```python
from build123d import *

# Parameters (mm, degrees)
SKETCH3_W                = 30
SKETCH3_H                = 25
BASETOPPLANE_DEPTH       = 30
BOSS_EXTRUDE1_DEPTH      = 5
BOSS_EXTRUDE1_DEPTH_BACK = 27
SKETCH6_W                = 34
SKETCH6_H                = 20
CUT_EXTRUDE1_DEPTH       = 39.668462602
SKETCH7_W                = 15
SKETCH7_H                = 10
BACKBAR_DEPTH            = 60
SIDECONNECT_DEPTH        = 5
SIDECONNECT_DEPTH_BACK   = 17
SKETCH8_W                = 40
SKETCH8_H                = 15
SKETCH9_W                = 30
SKETCH9_H                = 25
SIDESLIDER_DEPTH         = 17.5
MOUNTINGCUT_DEPTH        = 88.316641384
DRILLFORMOVEMENT_D       = 10
SKETCH17_W               = 15
SKETCH17_H               = 15
FRONTBAR_DEPTH           = 50


with BuildPart() as part:
    # Sketch3 → baseTopPlane (new body)
    with BuildSketch(Plane(origin=(0, 0, 0), x_dir=(1, 0, 0), z_dir=(0, 1, 0))):
        Rectangle(SKETCH3_W, SKETCH3_H)
    extrude(amount=BASETOPPLANE_DEPTH)

    # Sketch6 → Boss-Extrude1 (add, two sides: drawn at the far end of the back side and taken through both)
    with BuildSketch(Plane.XY.offset(12.5).offset(-BOSS_EXTRUDE1_DEPTH_BACK)):
        with Locations((0, 14.294511799)):
            Rectangle(SKETCH6_W, SKETCH6_H)
    extrude(amount=BOSS_EXTRUDE1_DEPTH + BOSS_EXTRUDE1_DEPTH_BACK)

    # Sketch4 → Cut-Extrude1 (cut, through all)
    with BuildSketch(Plane(origin=(0, 30, 0), x_dir=(1, 0, 0), z_dir=(0, 1, 0))):
        with BuildLine():
            Line((0, -12.5), (10, -12.5))
            Line((10, -12.5), (8, -10.5))
            Line((8, -10.5), (8, -8.5))
            ThreePointArc((8, -8.5), (9.060660172, -8.060660172), (9.5, -7))
            ThreePointArc((9.5, -7), (9.646446609, -6.646446609), (10, -6.5))
            Line((10, -6.5), (10, -4.5))
            ThreePointArc((10, -4.5), (8.939339828, -4.060660172), (8.5, -3))
            ThreePointArc((8.5, -3), (8.353553391, -2.646446609), (8, -2.5))
            Line((8, -2.5), (0, -2.5))
            Line((0, -2.5), (0, -12.5))
        make_face()
    cut_extrude1 = extrude(amount=-CUT_EXTRUDE1_DEPTH, mode=Mode.SUBTRACT)

    # Mirror1: Cut-Extrude1 across plane
    add(cut_extrude1.mirror(Plane(origin=(0, 0, 2.5), x_dir=(0, 0, 1), z_dir=(-1, 0, 0))), mode=Mode.SUBTRACT)

    # Sketch7 → BackBar (add)
    with BuildSketch(Plane(origin=(0, 0, -14.5), x_dir=(-1, 0, 0), z_dir=(0, 0, -1))):
        with Locations((0, 14.294511799)):
            Rectangle(SKETCH7_W, SKETCH7_H)
    extrude(amount=BACKBAR_DEPTH)

    # Sketch8 → sideConnect (add, two sides: drawn at the far end of the back side and taken through both)
    with BuildSketch(Plane.ZY.offset(7.5).offset(-SIDECONNECT_DEPTH_BACK)):
        with Locations((-57.5, 14.294511799)):
            Rectangle(SKETCH8_W, SKETCH8_H)
    extrude(amount=SIDECONNECT_DEPTH + SIDECONNECT_DEPTH_BACK)

    # Sketch9 → sideSlider (add)
    with BuildSketch(Plane.ZY.offset(12.5)):
        with Locations((-57.5, 14.294511799)):
            Rectangle(SKETCH9_W, SKETCH9_H)
    extrude(amount=SIDESLIDER_DEPTH)

    # Sketch13 → mountingCut (cut, through all)
    with BuildSketch(Plane(origin=(0, 26.794511799, 0), x_dir=(1, 0, 0), z_dir=(0, 1, 0))):
        Polygon((-30, 64), (-30, 51), (-24.75, 51), (-23.5, 49.75), (-26.25, 49.75), (-26.25, 47.25), (-19.75, 47.25), (-19.75, 53.75), (-22.25, 53.75), (-22.25, 51.25), (-24.75, 53.75), (-24.75, 61.25), (-22.25, 63.75), (-22.25, 61.25), (-19.75, 61.25), (-19.75, 67.75), (-26.25, 67.75), (-26.25, 65.25), (-23.5, 65.25), (-24.75, 64), align=None)
    extrude(amount=-MOUNTINGCUT_DEPTH, mode=Mode.SUBTRACT)

    # DrillforMovement (through all)
    with Locations(Plane(origin=(0, 21.794511799, 0), x_dir=(1, 0, 0), z_dir=(0, 1, 0))):
        with Locations((0, 57.5)):
            Hole(DRILLFORMOVEMENT_D / 2)

    # Sketch17 → frontBar (add)
    with BuildSketch(Plane.XY.offset(17.5)):
        with Locations((0, 14.294511799)):
            Rectangle(SKETCH17_W, SKETCH17_H)
    extrude(amount=FRONTBAR_DEPTH)


solid = part.part
```
Here's how the part is built. I have some questions about the finished solid (model axes, mm). A direction names the side the tool comes from. Give positions to 0.01 mm unless a question says otherwise; leave off trailing zeros. Loops run counter-clockwise (first coordinate to the right, second up) from the corner with the lowest first, then second, coordinate; pieces in that order, holes last. Notation, with made-up numbers: M 37,22 L 41,22 A26 cw 41,49 Z; hole C 53.25,69.25 d4. An arc over 180 degrees is marked long. Return JSON: item names as keys, results as strings.
Item 1: On a 3-axis mill with a long thin cutter (end or side, diameter ignored), from which of +Z, -Z, +X, -X, +Y, -Y can I reach the whole of each face in a straight line? I mean faces 1 (the flat face through (0, 19.295, -26)), 2 (the flat face through (-27, 14, -51)), 3 (the flat face through (-6, 6.795, -58)), 4 (the flat face through (-19.75, 14, -50)). Say none if no direction works.
A:
{"face 1": "+X, -X, +Y", "face 2": "-X, +Y, -Y", "face 3": "-Z, +X, -Y", "face 4": "+Y, -Y"}
Item 2: Thinking about a two-plate mould opening in X: for faces 5 (the flat face through (12, 27, 12.5)), 6 (the flat face through (15, 27, 0)), 7 (the flat face through (-26.25, 14, -49)), 8 (the flat face through (-30, 14, -68)), which applies, released by +X, released by -X, zero draft, split by the parting line, or undercut?
A:
{"face 5": "zero draft", "face 6": "released by +X", "face 7": "undercut", "face 8": "released by -X"}
Item 3: I'm going to push flat-ended pins straight in: pin 1 Ø3.5 at (y, z) = (2.5, -4) entering from +X; pin 2 Ø1.5 at (x, y) = (12, 15.5) entering from -Z; pin 3 Ø7.5 at (x, z) = (3.5, 52) entering from -Y. Where does each tip first touch, or does it pass through?
A:
{"pin 1": "stops at x = 15", "pin 2": "stops at z = -14.5", "pin 3": "stops at y = 6.79"}
Item 4: Imagine slicing it at C-C on z = -3.5. List the corners of the cut face in (x, y) for me.
A:
{"outline": "M -17,4.29 L -15,4.29 L -15,0 L 15,0 L 15,4.29 L 17,4.29 L 17,24.29 L 15,24.29 L 15,30 L -15,30 L -15,24.29 L -17,24.29 Z"}
Item 5: Imagine slicing it at B-B on x = 0. List the corners of the cut face in (y, z) for me, then the cut area to 3 significant figures.
A:
{"outline": "M 0,-12.5 L 4.29,-12.5 L 4.29,-14.5 L 9.29,-14.5 L 9.29,-37.5 L 6.79,-37.5 L 6.79,-52.5 L 21.79,-52.5 L 21.79,-37.5 L 19.29,-37.5 L 19.29,-14.5 L 24.29,-14.5 L 24.29,-12.5 L 30,-12.5 L 30,2.5 L 0,2.5 Z; M 4.29,12.5 L 24.29,12.5 L 24.29,17.5 L 21.79,17.5 L 21.79,67.5 L 6.79,67.5 L 6.79,17.5 L 4.29,17.5 Z; M 6.79,-77.5 L 21.79,-77.5 L 21.79,-62.5 L 6.79,-62.5 Z", "area": "2,020 mm^2"}
Item 6: Please list where these lines run through material, in increasing order: line 1 (Z direction, x = 0, y = 11); line 2 (Z direction, x = -20.5, y = 25); line 3 (X direction, y = 10, z = -57.5).
A:
{"line 1": "z = -77.5 to -62.5, -52.5 to 2.5, 12.5 to 67.5", "line 2": "z = -72.5 to -67.75, -61.25 to -53.75, -47.25 to -42.5", "line 3": "x = -24.75 to -5, 5 to 9.5"}
Item 7: Imagine slicing it at D-D on z = 41. List the corners of the cut face in (x, y) for me.
A:
{"outline": "M -7.5,6.79 L 7.5,6.79 L 7.5,21.79 L -7.5,21.79 Z"}
Item 8: Imagine slicing it at A-A on z = -57.5. List the corners of the cut face in (x, y) for me, then the cut area to 3 significant figures.
A:
{"outline": "M -24.75,1.79 L -12.5,1.79 L -12.5,6.79 L -5,6.79 L -5,21.79 L -12.5,21.79 L -12.5,26.79 L -24.75,26.79 Z; M 5,6.79 L 9.5,6.79 L 9.5,21.79 L 5,21.79 Z", "area": "486 mm^2"}
